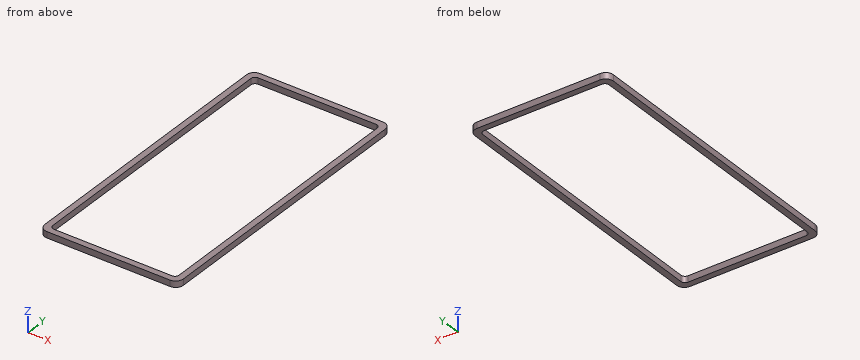
from build123d import *

# Parameters (mm, degrees)
ESQUISSE1_W        = 900
ESQUISSE1_H        = 1900
ESQUISSE1_W_2      = 820
ESQUISSE1_H_2      = 1820
BOSS_EXTRU_1_DEPTH = 40
CONG_1_R           = 50
CONG_2_R           = 25


with BuildPart() as part:
    # Esquisse1 → Boss.-Extru.1 (new body)
    with BuildSketch(Plane.XY):
        with Locations((450, 950)):
            Rectangle(ESQUISSE1_W, ESQUISSE1_H)
        with Locations((450, 950)):
            Rectangle(ESQUISSE1_W_2, ESQUISSE1_H_2, mode=Mode.SUBTRACT)
    extrude(amount=BOSS_EXTRU_1_DEPTH)

    # Congé1
    cong_1_edges = [part.edges().sort_by_distance(p)[0] for p in [
        (0, 1900, 20),
        (900, 1900, 20),
        (900, 0, 20),
        (0, 0, 20),
    ]]
    fillet(cong_1_edges, radius=CONG_1_R)

    # Congé2
    cong_2_edges = [part.edges().sort_by_distance(p)[0] for p in [
        (40, 1860, 20),
        (40, 40, 20),
        (860, 40, 20),
        (860, 1860, 20),
    ]]
    fillet(cong_2_edges, radius=CONG_2_R)


solid = part.part
The listing builds one solid part. Answer for the finished solid, in the listing's coordinates (mm). Round coordinates to 2 decimals unless told otherwise and drop trailing zeros. Order: outer loops, then holes, each group sorted by start corner. A loop starts at its lowest first (then second) coordinate and runs counter-clockwise, first axis right, second up. Notation, with made-up numbers: (-37, 45.5) -> (-1, 45.5) arc R25 ccw to (-1, 80.5) -> close; hole circle Ø1 at (74.5, -25). An arc over 180 degrees is marked (long way). Put each result on its own line as item: value.
Q1. Section C-C, the plane y = 1137.5 is taken. Write down the section's boundary in (x, z), and give its area (3 significant figures).
Results list:
outline: (0, 0) -> (40, 0) -> (40, 40) -> (0, 40) -> close; (860, 0) -> (900, 0) -> (900, 40) -> (860, 40) -> close
area: 3,200 mm^2
Q2. Section A-A, the plane x = 814 is taken. Write down the section's boundary in (y, z).
Results list:
outline: (0, 0) -> (40, 0) -> (40, 40) -> (0, 40) -> close; (1860, 0) -> (1900, 0) -> (1900, 40) -> (1860, 40) -> close
Q3. Consider line 1 along Y through (x, z) = (292.5, 31.5); line 2 along X through (y, z) = (198.5, 33). Determine where each line is inside the solid, lowest interval first.
Results list:
line 1: 0 to 40, 1860 to 1900
line 2: 0 to 40, 860 to 900
Q4. Section B-B, the plane z = 15 is taken. Write down the section's boundary in (x, y), and give its area (3 significant figures).
Results list:
outline: (0, 50) arc R50 ccw to (50, 0) -> (850, 0) arc R50 ccw to (900, 50) -> (900, 1850) arc R50 ccw to (850, 1900) -> (50, 1900) arc R50 ccw to (0, 1850) -> close; hole (40, 65) arc R25 ccw to (65, 40) -> (835, 40) arc R25 ccw to (860, 65) -> (860, 1835) arc R25 ccw to (835, 1860) -> (65, 1860) arc R25 ccw to (40, 1835) -> close
area: 216,000 mm^2
